The listing builds one solid part. Answer for the finished solid, in the listing's coordinates (mm). A direction names the side the tool comes from. Round coordinates to 2 decimals unless told otherwise and drop trailing zeros. Write each loop counter-clockwise with the first axis right and the second up, starting at its lowest first coordinate (ties: lowest second). Pieces come first, ordered by that corner, then holes. Notation, with made-up numbers: (11, 10) - (64, 10) arc R27 cw to (64, 40) - close; hole circle Ø5 at (42, 44.25). An arc over 180 degrees is marked (long way). Answer in a Markdown table with one row per item.
from build123d import *

# Parameters (mm, degrees)
F1_DEPTH  = 55
F2_R      = 4
F3_DEPTH  = 29.3
F5_DEPTH  = 33.2
F7_DEPTH  = 34.5
F1_FACE_R = 3.3
F9_DEPTH  = 37.2


with BuildPart() as f1:
    # F0 (on Top) → F1 (new body)
    with BuildSketch(Plane.XY):
        with BuildLine():
            Line((58.593456, -9.011728), (58.593456, 55.988272))
            Line((58.593456, 55.988272), (38.093456, 55.988272))
            Line((38.093456, 55.988272), (38.093456, 36.488272))
            Line((38.093456, 36.488272), (12.593456, 36.488272))
            Line((12.593456, 36.488272), (12.593456, 24.488272))
            Line((12.593456, 24.488272), (28.160421, 24.488272))
            ThreePointArc((28.160421, 24.488272), (43.093456, 23.488272), (28.160421, 22.488272))
            Line((28.160421, 22.488272), (12.593456, 22.488272))
            Line((12.593456, 22.488272), (12.593456, 10.488272))
            Line((12.593456, 10.488272), (38.093456, 10.488272))
            Line((38.093456, 10.488272), (38.093456, -9.011728))
            Line((38.093456, -9.011728), (58.593456, -9.011728))
        make_face()
    extrude(amount=F1_DEPTH)

    # F2 (on face) → F3 (cut)
    with BuildSketch(Plane(origin=(0, 36.488272, 0), x_dir=(-1, 0, 0), z_dir=(0, 1, 0))):
        with Locations((-21.593456, 10)):
            Circle(F2_R)
        with BuildLine():
            ThreePointArc((-17.593456, 45), (-18.765028, 47.828427), (-21.593456, 49))
            ThreePointArc((-21.593456, 49), (-24.421883, 42.171573), (-17.593456, 45))
        make_face()
    extrude(amount=-F3_DEPTH, mode=Mode.SUBTRACT)

    # F4 (on face) → F5 (cut)
    with BuildSketch(Plane(origin=(38.093456, 0, 0), x_dir=(0, -1, 0), z_dir=(-1, 0, 0))):
        with BuildLine():
            ThreePointArc((3.3, 45), (2.333452, 47.333452), (0, 48.3))
            ThreePointArc((0, 48.3), (-2.333452, 42.666548), (3.3, 45))
        make_face()
        with BuildLine():
            ThreePointArc((3.3, 10), (-2.333452, 12.333452), (0, 6.7))
            ThreePointArc((0, 6.7), (2.333452, 7.666548), (3.3, 10))
        make_face()
    extrude(amount=-F5_DEPTH, mode=Mode.SUBTRACT)

    # F6 (on face) → F7 (cut)
    with BuildSketch(Plane(origin=(38.093456, 0, 0), x_dir=(0, -1, 0), z_dir=(-1, 0, 0))):
        with BuildLine():
            ThreePointArc((-42.938272, 45), (-43.90482, 47.333452), (-46.238272, 48.3))
            ThreePointArc((-46.238272, 48.3), (-48.571725, 42.666548), (-42.938272, 45))
        make_face()
    extrude(amount=-F7_DEPTH, mode=Mode.SUBTRACT)

    # F8 (on face) + F1_face (on face) → F9 (cut)
    with BuildSketch(Plane(origin=(38.093456, 0, 0), x_dir=(0, -1, 0), z_dir=(-1, 0, 0))):
        with BuildLine():
            ThreePointArc((-42.938272, 10), (-48.571725, 12.333452), (-46.238272, 6.7))
            ThreePointArc((-46.238272, 6.7), (-43.90482, 7.666548), (-42.938272, 10))
        make_face()
    with BuildSketch(Plane(origin=(25.343456, 36.488272, 27.5), x_dir=(-1, 0, 0), z_dir=(0, 1, 0))):
        Polygon((-33.25, 27.5), (-33.25, -27.5), (-33.25, -27.5), (-33.25, 27.5), align=None)
        with Locations((-33.25, 17.5)):
            Circle(F1_FACE_R, mode=Mode.SUBTRACT)
        with Locations((-33.25, 17.5)):
            Circle(F1_FACE_R, mode=Mode.SUBTRACT)
        with Locations((-33.25, -17.5)):
            Circle(F1_FACE_R, mode=Mode.SUBTRACT)
    extrude(amount=-F9_DEPTH, mode=Mode.SUBTRACT)


solid = f1.part
(1) Section C-C (y = 33.5) is taken. Give the vertices of the cut face in (x, z).
Checked values:
| item | result |
|---|---|
| outline | (12.59, 0) - (58.59, 0) - (58.59, 55) - (12.59, 55) - close; hole circle Ø8 at (21.59, 10); hole (17.59, 45) arc R4 ccw (long way) to (21.59, 49) arc R4 ccw to start |
(2) For faces 1 (the flat face through (20, 24.488, 27)), 2 (the flat face through (48, 55.988, 27)), 3 (the flat face through (38.093, 46, 27)), 4 (the flat face through (25, 10.488, 27)), determine the directions among +Z, -Z, +X, -X, +Y, -Y from which every point of the face is accessible in a straight line to the end or side of a thin tool.
Checked values:
| item | result |
|---|---|
| face 1 | +Z, -Z, -X |
| face 2 | +Z, -Z, +X, -X, +Y |
| face 3 | +Z, -Z, -X, +Y |
| face 4 | +Z, -Z, -X, -Y |
(3) Section B-B (z = 46) is taken. Give the vertices of the cut face in (x, y).
Checked values:
| item | result |
|---|---|
| outline | (12.59, 10.49) - (17.72, 10.49) - (17.72, 22.49) - (12.59, 22.49) - close; (12.59, 24.49) - (17.72, 24.49) - (17.72, 36.49) - (12.59, 36.49) - close; (25.47, 10.49) - (38.09, 10.49) - (38.09, 3.14) - (58.59, 3.14) - (58.59, 43.09) - (38.09, 43.09) - (38.09, 36.49) - (25.47, 36.49) - (25.47, 24.49) - (28.16, 24.49) arc R7.5 cw (long way) to (28.16, 22.49) - (25.47, 22.49) - close; (38.09, -9.01) - (58.59, -9.01) - (58.59, -3.14) - (38.09, -3.14) - close; (38.09, 49.38) - (58.59, 49.38) - (58.59, 55.99) - (38.09, 55.99) - close |
(4) Section A-A (x = 46) is taken. Give the vertices of the cut face in (y, z).
Checked values:
| item | result |
|---|---|
| outline | (-9.01, 0) - (55.99, 0) - (55.99, 55) - (-9.01, 55) - close; hole (-3.3, 10) arc R3.3 ccw to (0, 6.7) arc R3.3 ccw (long way) to start; hole (-3.3, 45) arc R3.3 ccw (long way) to (0, 48.3) arc R3.3 ccw to start; hole (42.94, 10) arc R3.3 ccw to (46.24, 6.7) arc R3.3 ccw (long way) to start; hole (42.94, 45) arc R3.3 ccw (long way) to (46.24, 48.3) arc R3.3 ccw to start |
(5) For a pull along Z with two mould halves and no side action, classify faces 5 (the flat face through (45, 24, 0)), 6 (the flat face through (26, 36.488, 27)), 7 (the cylindrical face through (17.778, 16.572, 11.201)) as pulls with the +Z half, pulls with the -Z half, needs draft (parallel to the pull), parting line crosses it, or undercut.
Checked values:
| item | result |
|---|---|
| face 5 | pulls with the -Z half |
| face 6 | needs draft |
| face 7 | undercut |
(6) Section D-D (z = 35) is taken. Give the vertices of the cut face in (x, y), and give its area (3 significant figures).
Checked values:
| item | result |
|---|---|
| outline | (12.59, 10.49) - (38.09, 10.49) - (38.09, -9.01) - (58.59, -9.01) - (58.59, 55.99) - (38.09, 55.99) - (38.09, 36.49) - (12.59, 36.49) - (12.59, 24.49) - (28.16, 24.49) arc R7.5 cw (long way) to (28.16, 22.49) - (12.59, 22.49) - close |
| area | 1,790 mm2 |
(7) Find the intervals of material crossed by line 1 (Y direction, x = 44.25, z = 45); line 2 (Y direction, x = 27, z = 30); line 3 (X direction, y = 2, z = 31.5), in increasing order.
Checked values:
| item | result |
|---|---|
| line 1 | y = -9.01 to -3.3, 3.3 to 42.94, 49.54 to 55.99 |
| line 2 | y = 10.49 to 22.49, 24.49 to 36.49 |
| line 3 | x = 38.09 to 58.59 |
(8) Flat-ended cylindrical pins translate along their axes: pin 1 (7 mm diameter, centred on x = 21.59, z = 45, fed in from -Y); pin 2 (13 mm diameter, centred on x = 30.5, z = 32, fed in from +Y); pin 3 (8.5 mm diameter, centred on y = 46.24, z = 10, fed in from -X); pin 4 (17 mm diameter, centred on x = 18.5, z = 36.5, fed in from -Y). Find the tip coordinate at first contact, or state that the pin passes through.
Checked values:
| item | result |
|---|---|
| pin 1 | passes through |
| pin 2 | stops at y = 36.49 |
| pin 3 | stops at x = 38.09 |
| pin 4 | stops at y = 10.49 |
